from build123d import *

# Parameters (mm, degrees)
BASE_FLANGE1_DEPTH         = 3.175
F_5_2_5_2_DIAMETER_HOLE1_D = 5.2


# Sheet-metal steps are written as plain solids
with BuildPart() as part:
    # Sketch11 → Base-Flange1 (new body)
    with BuildSketch(Plane.XY.offset(423.175)):
        with BuildLine():
            Line((80.932869831, 272.193100025), (72.492212082, 320.048916024))
            ThreePointArc((72.492212082, 320.048916024), (65.651606735, 331.8961997), (52.796224992, 336.575))
            Line((52.796224992, 336.575), (20, 336.575))
            Line((20, 336.575), (20, 359))
            ThreePointArc((20, 359), (19.707106781, 359.707106781), (19, 360))
            Line((19, 360), (1, 360))
            ThreePointArc((1, 360), (0.292893219, 359.707106781), (0, 359))
            Line((0, 359), (0, 308))
            ThreePointArc((0, 308), (2.928932188, 300.928932188), (10, 298))
            Line((10, 298), (39.289001969, 298))
            ThreePointArc((39.289001969, 298), (52.143642752, 293.321821378), (58.984652965, 281.475821034))
            Line((58.984652965, 281.475821034), (61.236098321, 268.718063502))
            ThreePointArc((61.236098321, 268.718063502), (65.348951759, 262.263898856), (72.820881831, 260.607980474))
            ThreePointArc((72.820881831, 260.607980474), (79.276674092, 264.720773785), (80.932869831, 272.193100025))
        make_face()
    extrude(amount=-BASE_FLANGE1_DEPTH)

    # Ø5.2 (5.2) Diameter Hole1 (through all)
    with Locations(Plane.XY.offset(423.175)):
        with Locations((67.610960265, 290.15212908), (10, 349.9999998), (10, 328.3784093), (10, 306.7568188), (71.083923819, 270.455974019)):
            Hole(F_5_2_5_2_DIAMETER_HOLE1_D / 2)


solid = part.part
Work out the finished part from the listing and answer in its coordinate system (mm). A direction names the side the tool comes from. Give positions to 0.01 mm unless a question says otherwise; leave off trailing zeros. Loops run counter-clockwise (first coordinate to the right, second up) from the corner with the lowest first, then second, coordinate; pieces in that order, holes last. Notation, with made-up numbers: (-35, 85.5) -> (17, 85.5) arc R22 ccw to (17, 91.5) -> close; hole circle Ø6 at (56, 32). An arc over 180 degrees is marked (long way). Use a Markdown table: item, result. Add a question column.
1. Section B-B on z = 421.7 is taken. Determine the outline of the cut face in (x, y) (3 decimals), and give its area (3 significant figures).
2. For faces 1 (the flat face through (60.095, 275.186, 421.61)), 2 (the flat face through (37, 336.575, 422)), determine the directions among +Z, -Z, +X, -X, +Y, -Y from which every point of the face is accessible in a straight line to the end or side of a thin tool.
3. Section C-C on x = 25 is taken. Determine the outline of the cut face in (y, z) (3 decimals).
4. Determine the mould class of faces 3 (the flat face through (20, 348, 422)), 4 (the cylindrical face through (10.338, 330.956, 421.565)), 5 (the flat face through (24, 298, 422)) for opening direction X: released by +X, released by -X, zero draft, split by the parting line, or undercut.
5. Section A-A on y = 350 is taken. Determine the outline of the cut face in (x, z) (3 decimals).
6. Flat-ended cylindrical pins translate along their axes: pin 1 Ø1.6 at (x, z) = (22.5, 421.5) entering from -Y; pin 2 Ø1 at (y, z) = (352, 421.5) entering from +X. Find the tip coordinate at first contact, or state that the pin passes through.
7. Find the intervals of material crossed by probe 1 along Y at (x, z) = (10, 422.5); probe 2 along Y at (x, z) = (69.5, 420.75); probe 3 along X at (y, z) = (341, 422.5), in increasing order.
8. Section D-D on y = 323 is taken. Determine the outline of the cut face in (x, z) (3 decimals), and give its area (3 significant figures).
Results below:
| question | item | result |
|---|---|---|
| 1 | outline | (0, 308) arc R10 ccw to (10, 298) -> (39.289, 298) arc R20 cw to (58.985, 281.476) -> (61.236, 268.718) arc R10 ccw to (72.821, 260.608) arc R10 ccw to (80.933, 272.193) -> (72.492, 320.049) arc R20 ccw to (52.796, 336.575) -> (20, 336.575) -> (20, 359) arc R1 ccw to (19, 360) -> (1, 360) arc R1 ccw to (0, 359) -> close; hole circle Ø5.2 at (10, 306.757); hole circle Ø5.2 at (10, 328.378); hole circle Ø5.2 at (10, 350); hole circle Ø5.2 at (67.611, 290.152); hole circle Ø5.2 at (71.084, 270.456) |
| 1 | area | 3,870 mm^2 |
| 2 | face 1 | +Z, -Z, -X, -Y |
| 2 | face 2 | +Z, -Z, +X, +Y |
| 3 | outline | (298, 420) -> (336.575, 420) -> (336.575, 423.175) -> (298, 423.175) -> close |
| 4 | face 3 | released by +X |
| 4 | face 4 | undercut |
| 4 | face 5 | zero draft |
| 5 | outline | (0, 420) -> (7.4, 420) -> (7.4, 423.175) -> (0, 423.175) -> close; (12.6, 420) -> (20, 420) -> (20, 423.175) -> (12.6, 423.175) -> close |
| 6 | pin 1 | stops at y = 298 |
| 6 | pin 2 | stops at x = 20 |
| 7 | probe 1 | y = 298 to 304.16, 309.36 to 325.78, 330.98 to 347.4, 352.6 to 360 |
| 7 | probe 2 | y = 260.58 to 268.39, 272.52 to 288.37, 291.94 to 327.57 |
| 7 | probe 3 | x = 0 to 20 |
| 8 | outline | (0, 420) -> (71.736, 420) -> (71.736, 423.175) -> (0, 423.175) -> close |
| 8 | area | 228 mm^2 |
